Can you work these out from the model? Positions are in its coordinate system, mm. A direction names the side the tool comes from. Give positions to 0.01 mm unless a question says otherwise; leave off trailing zeros. Order: outer loops, then holes, each group sorted by start corner. A loop starts at its lowest first (then second) coordinate and runs counter-clockwise, first axis right, second up. Notation, with made-up numbers: (-38, -4) -> (-7, -4) arc R9 cw to (-7, 0) -> close; hole circle Ø1 at (-32.75, 60.25). An arc over 180 degrees is marked (long way). Answer as a JSON object with one key per item and string values.
```python
from build123d import *

# Parameters (mm, degrees)
CROQUIS1_R                   = 55
DISCO_DEPTH                  = 5
CORTAR_EXTRUIR1_DEPTH        = 10
SALIENTE_EXTRUIR1_DEPTH      = 10
SALIENTE_EXTRUIR1_DEPTH_BACK = 5
CROQUIS7_R                   = 60
CROQUIS7_R_2                 = 55
CROQUIS7_R_3                 = 53
SALIENTE_EXTRUIR6_DEPTH      = 5
CROQUIS9_R                   = 1.5875
CORTAR_EXTRUIR2_DEPTH        = 87.168439698
CROQUIS10_R                  = 3
CORTAR_EXTRUIR3_DEPTH        = 3


with BuildPart() as part:
    # Croquis1 → Disco (new body)
    with BuildSketch(Plane.XY):
        Circle(CROQUIS1_R)
    extrude(amount=DISCO_DEPTH)

    # Croquis6 → Cortar-Extruir1 (cut)
    with BuildSketch(Plane.XY.offset(5)):
        with BuildLine():
            Line((-5.25, 0), (-5.25, -30))
            ThreePointArc((-5.25, -30), (0, -35.25), (5.25, -30))
            Line((5.25, -30), (5.25, 0))
            ThreePointArc((5.25, 0), (0, 5.25), (-5.25, 0))
        make_face()
        with BuildLine():
            Line((2.625, 4.54663337), (-23.355762114, 19.54663337))
            ThreePointArc((-23.355762114, 19.54663337), (-30.527395483, 17.625), (-28.605762114, 10.45336663))
            Line((-28.605762114, 10.45336663), (-2.625, -4.54663337))
            ThreePointArc((-2.625, -4.54663337), (4.54663337, -2.625), (2.625, 4.54663337))
        make_face()
        with BuildLine():
            Line((2.625, -4.54663337), (28.605762114, 10.45336663))
            ThreePointArc((28.605762114, 10.45336663), (30.527395483, 17.625), (23.355762114, 19.54663337))
            Line((23.355762114, 19.54663337), (-2.625, 4.54663337))
            ThreePointArc((-2.625, 4.54663337), (-4.54663337, -2.625), (2.625, -4.54663337))
        make_face()
    extrude(amount=-CORTAR_EXTRUIR1_DEPTH, mode=Mode.SUBTRACT)

    # Croquis7 → Saliente-Extruir1 (add, two sides: drawn at the far end of the back side and taken through both)
    # profile 1 of 2: a face of its own
    with BuildSketch(Plane.XY.offset(5).offset(-SALIENTE_EXTRUIR1_DEPTH_BACK)):
        Circle(CROQUIS7_R)
        Circle(CROQUIS7_R_2, mode=Mode.SUBTRACT)
    # profile 2 of 2: a face of its own
    with BuildSketch(Plane.XY.offset(5).offset(-SALIENTE_EXTRUIR1_DEPTH_BACK)):
        Circle(CROQUIS7_R_2)
        Circle(CROQUIS7_R_3, mode=Mode.SUBTRACT)
    extrude(amount=SALIENTE_EXTRUIR1_DEPTH + SALIENTE_EXTRUIR1_DEPTH_BACK)

    # Croquis8 → Saliente-Extruir6 (add)
    with BuildSketch(Plane.XY.offset(5)):
        Polygon((-8.714101615, -5.031088913), (0, 10.062177826), (8.714101615, -5.031088913), align=None)
    extrude(amount=-SALIENTE_EXTRUIR6_DEPTH)

    # Croquis9 → Cortar-Extruir2 (cut, through all)
    with BuildSketch(Plane.XY.offset(15)):
        with Locations((0, 55.5)):
            Circle(CROQUIS9_R)
        with Locations((48.06440991, -27.75)):
            Circle(CROQUIS9_R)
        with Locations((-48.06440991, -27.75)):
            Circle(CROQUIS9_R)
    extrude(amount=-CORTAR_EXTRUIR2_DEPTH, mode=Mode.SUBTRACT)

    # Croquis10 → Cortar-Extruir3 (cut)
    with BuildSketch(Plane(origin=(0, 0, 0), x_dir=(-1, 0, 0), z_dir=(0, 0, -1))):
        with Locations((0, 55.5)):
            Circle(CROQUIS10_R)
        with Locations((48.06440991, -27.75)):
            Circle(CROQUIS10_R)
        with Locations((-48.06440991, -27.75)):
            Circle(CROQUIS10_R)
    extrude(amount=-CORTAR_EXTRUIR3_DEPTH, mode=Mode.SUBTRACT)


solid = part.part
```
1. Please list where these lines run through material, in increasing order: L1, parallel to Y at x = 0, z = 11.5; L2, parallel to Y at x = 0, z = 2.05; L3, parallel to X at y = 14.5, z = 4.75.
Worked answers:
{"L1": "-60 to -53, 53 to 53.91, 57.09 to 60", "L2": "-60 to -35.25, -5.03 to 52.5, 58.5 to 60", "L3": "-58.22 to -31.21, -14.61 to 14.61, 31.21 to 58.22"}
2. If we section it at A-A on x = 0: Please give me the cut outline in (y, z).
Worked answers:
{"outline": "(-60, 0) -> (-35.25, 0) -> (-35.25, 5) -> (-53, 5) -> (-53, 15) -> (-60, 15) -> close; (-5.03, 0) -> (52.5, 0) -> (52.5, 3) -> (53.91, 3) -> (53.91, 15) -> (53, 15) -> (53, 5) -> (-5.03, 5) -> close; (57.09, 3) -> (58.5, 3) -> (58.5, 0) -> (60, 0) -> (60, 15) -> (57.09, 15) -> close"}
3. For faces 3 (the face through (5.25, -18, 3)), 4 (the face through (28, 45, 10)), 5 (the face through (51.06, -27.62, 1.48)), which set-ups out of +Z, -Z, +X, -X, +Y, -Y let a thin tool reach every point of the face, with its end or its side?
Worked answers:
{"face 3": "+Z, -Z", "face 4": "+Z", "face 5": "-Z"}
4. If we section it at D-D on x = 13.5: Please give me the cut outline in (y, z), then the cut area to 3 significant figures.
Worked answers:
{"outline": "(-58.46, 0) -> (1.73, 0) -> (1.73, 5) -> (-51.25, 5) -> (-51.25, 15) -> (-58.46, 15) -> close; (13.86, 0) -> (58.46, 0) -> (58.46, 15) -> (51.25, 15) -> (51.25, 5) -> (13.86, 5) -> close", "area": "668 mm²"}
5. If we mould it in two halves opening along Y, with no side actions, what happens to faces 1 (the face through (-0.207, 57.074, 9.084)), 2 (the face through (-1, 1, 0))? For each: +Y half, -Y half, draft (parallel to the pull), parting line (faces both ways), or undercut.
Worked answers:
{"face 1": "undercut", "face 2": "draft"}
6. Will these pins go through, and if not, where does the flat tip stop? pin 1 Ø5 at (x, y) = (-48.06, -27.75) entering from -Z; pin 2 Ø1.5 at (x, y) = (-21, -14.5) entering from +Z; pin 3 Ø2.5 at (x, z) = (-2, 2) entering from -Y.
Worked answers:
{"pin 1": "z = 3", "pin 2": "z = 5", "pin 3": "y = -60"}
7. If we section it at C-C on z = 13: Count the separate pieces of the cut face and the enclosed holes in it, then the cut area to 3 significant figures.
Worked answers:
{"separate pieces": "1", "enclosed holes": "4", "area": "2,460 mm²"}
8. If we section it at B-B on y = 55.5: Please give me the cut outline in (x, z), then the cut area to 3 significant figures.
Worked answers:
{"outline": "(-22.8, 0) -> (-3, 0) -> (-3, 3) -> (-1.59, 3) -> (-1.59, 15) -> (-22.8, 15) -> close; (1.59, 3) -> (3, 3) -> (3, 0) -> (22.8, 0) -> (22.8, 15) -> (1.59, 15) -> close", "area": "628 mm²"}
